from build123d import *

# Parameters (mm, degrees)
SURFACE_EXTRUDE2_1_DEPTH = 115
THICKEN3_T2              = 2
BOSS_EXTRUDE2_REACH      = 890.848
SKETCH11_W               = 70
SKETCH11_H               = 115
BOSS_EXTRUDE7_DEPTH      = 2
SKETCH17_W               = 2.5
SKETCH17_H               = 115
BOSS_EXTRUDE8_DEPTH      = 15
SKETCH22_W               = 1.5
SKETCH22_H               = 105
CUT_EXTRUDE1_DEPTH       = 5
SKETCH23_W               = 64.9
SKETCH23_H               = 2
BOSS_EXTRUDE9_DEPTH      = 15
SKETCH25_W               = 64.9
SKETCH25_H               = 3.5
BOSS_EXTRUDE10_DEPTH     = 15
SKETCH26_W               = 20
SKETCH26_H               = 1.5
CUT_EXTRUDE3_DEPTH       = 15
SKETCH27_W               = 5
SKETCH27_H               = 9
CUT_EXTRUDE4_DEPTH       = 1.1
SKETCH29_W               = 2.5
SKETCH29_H               = 55
CUT_EXTRUDE6_DEPTH       = 1
CUT_EXTRUDE7_REACH       = 905.754
CUT_EXTRUDE7_END_RADIUS  = 63.3
SKETCH30_R               = 2.5
FILLET1_R                = 1
CUT_EXTRUDE8_REACH       = 909.037
SKETCH31_W               = 35
SKETCH31_H               = 3
CUT_EXTRUDE9_REACH       = 905.975
SKETCH32_R               = 1.5
SKETCH33_W               = 1.5
SKETCH33_H               = 5.890969975
BOSS_EXTRUDE11_DEPTH     = 1.5
MIRROR24_COPY_1_REACH    = 905.975
MIRROR24_COPY_1_SKETCH_R = 1.5


with BuildPart() as body_1:
    # Surface-Extrude2: a surface, the sketch's curves swept straight by 115 mm
    with BuildLine(Plane(origin=(0, 0, 0), x_dir=(1, 0, 0), z_dir=(0, 1, 0)), mode=Mode.PRIVATE) as surface_extrude2_1_path:
        ThreePointArc((-880.139667207, 63.554736355), (-845.139667207, 52.580574649), (-810.139667207, 63.554736355))
    surface_extrude2_1 = Shell.extrude(surface_extrude2_1_path.wire(), (0 * SURFACE_EXTRUDE2_1_DEPTH, 1 * SURFACE_EXTRUDE2_1_DEPTH, 0 * SURFACE_EXTRUDE2_1_DEPTH))
    add(Solid.thicken(surface_extrude2_1, -THICKEN3_T2))

    # Sketch11 → Boss-Extrude2 (add, up to next)
    with BuildSketch(Plane(origin=(0, 0, -63.554736355), x_dir=(-1, 0, 0), z_dir=(0, 0, -1)), mode=Mode.PRIVATE) as boss_extrude2_sk1:
        with Locations((845.139667207, 57.5)):
            Rectangle(SKETCH11_W, SKETCH11_H)
    boss_extrude2_tool1 = extrude(boss_extrude2_sk1.sketch, amount=-BOSS_EXTRUDE2_REACH, mode=Mode.PRIVATE) - body_1.part
    add(boss_extrude2_tool1.solids().sort_by_distance((-845.139667, 57.5, -63.554736))[0])

    # Sketch15 → Boss-Extrude7 (add)
    with BuildSketch(Plane(origin=(0, 0, -51.554736355), x_dir=(-1, 0, 0), z_dir=(0, 0, -1))):
        with BuildLine():
            Line((890.139667207, 24.998904399), (845.139667207, 24.998904399))
            Line((845.139667207, 24.998904399), (845.139667207, 15))
            Line((845.139667207, 15), (889.991644173, 15))
            ThreePointArc((889.991644173, 15), (895.139667207, 19.924336912), (890.139667207, 24.998904399))
        make_face()
        with BuildLine():
            Line((891.281592166, 100), (845.139667207, 100))
            Line((845.139667207, 100), (845.139667207, 90.00121851))
            Line((845.139667207, 90.00121851), (891.171212738, 90.00121851))
            ThreePointArc((891.171212738, 90.00121851), (896.281287529, 94.944806923), (891.281592166, 100))
        make_face()
    boss_extrude7 = extrude(amount=BOSS_EXTRUDE7_DEPTH)

    # Mirror20: Boss-Extrude7 across plane
    add(boss_extrude7.mirror(Plane.ZY.offset(845.139667207)))

    # Sketch17 → Boss-Extrude8 (add)
    with BuildSketch(Plane(origin=(0, 0, -63.554736355), x_dir=(-1, 0, 0), z_dir=(0, 0, -1))):
        with Locations((878.889667207, 57.5)):
            Rectangle(SKETCH17_W, SKETCH17_H)
        with Locations((811.489667207, 57.5)):
            Rectangle(SKETCH17_W, SKETCH17_H)
    extrude(amount=BOSS_EXTRUDE8_DEPTH)

    # Sketch22 → Cut-Extrude1 (cut)
    with BuildSketch(Plane(origin=(0, 0, -78.554736355), x_dir=(-1, 0, 0), z_dir=(0, 0, -1))):
        with Locations((811.989667207, 55.5)):
            Rectangle(SKETCH22_W, SKETCH22_H)
    cut_extrude1 = extrude(amount=-CUT_EXTRUDE1_DEPTH, mode=Mode.SUBTRACT)

    # Mirror21: Cut-Extrude1 across plane
    add(cut_extrude1.mirror(Plane.ZY.offset(845.139667207)), mode=Mode.SUBTRACT)

    # Sketch23 → Boss-Extrude9 (add)
    with BuildSketch(Plane(origin=(0, 0, -63.554736355), x_dir=(-1, 0, 0), z_dir=(0, 0, -1))):
        with Locations((845.189667207, 114)):
            Rectangle(SKETCH23_W, SKETCH23_H)
        with Locations((845.189667207, 110)):
            Rectangle(SKETCH23_W, SKETCH23_H)
    extrude(amount=BOSS_EXTRUDE9_DEPTH)

    # Sketch25 → Boss-Extrude10 (add)
    with BuildSketch(Plane(origin=(0, 0, -63.554736355), x_dir=(-1, 0, 0), z_dir=(0, 0, -1))):
        with Locations((845.189667207, 1.75)):
            Rectangle(SKETCH25_W, SKETCH25_H)
    extrude(amount=BOSS_EXTRUDE10_DEPTH)

    # Sketch26 → Cut-Extrude3 (cut)
    with BuildSketch(Plane(origin=(0, 0, -78.554736355), x_dir=(-1, 0, 0), z_dir=(0, 0, -1))):
        with Locations((825.239667207, 1.75)):
            Rectangle(SKETCH26_W, SKETCH26_H)
    extrude(amount=-CUT_EXTRUDE3_DEPTH, mode=Mode.SUBTRACT)

    # Sketch27 → Cut-Extrude4 (cut)
    with BuildSketch(Plane.ZY.offset(880.139667207)):
        with Locations((-75.146974965, 83)):
            Rectangle(SKETCH27_W, SKETCH27_H)
    extrude(amount=-CUT_EXTRUDE4_DEPTH, mode=Mode.SUBTRACT)

    # Sketch29 → Cut-Extrude6 (cut)
    with BuildSketch(Plane(origin=(-810.239667207, 0, 0), x_dir=(0, 0, -1), z_dir=(1, 0, 0))):
        with Locations((77.304736355, 35.5)):
            Rectangle(SKETCH29_W, SKETCH29_H)
    extrude(amount=-CUT_EXTRUDE6_DEPTH, mode=Mode.SUBTRACT)

    # Cut-Extrude7: up to this cylinder (the profile starts inside it)
    cut_extrude7_end = Plane(origin=(-845.139667207, 104, -113.880574649), z_dir=(0, 1, 0)) * Cylinder(CUT_EXTRUDE7_END_RADIUS, 1939.108, mode=Mode.PRIVATE)
    # Sketch30 → Cut-Extrude7 (cut, up to the surface)
    with BuildSketch(Plane(origin=(0, 0, -63.554736355), x_dir=(-1, 0, 0), z_dir=(0, 0, -1)), mode=Mode.PRIVATE) as cut_extrude7_sk1:
        with Locations((822.739667207, 104)):
            Circle(SKETCH30_R)
    cut_extrude7_tool1 = extrude(cut_extrude7_sk1.sketch, amount=-CUT_EXTRUDE7_REACH, mode=Mode.PRIVATE) & cut_extrude7_end
    add(cut_extrude7_tool1.solids().sort_by_distance((-822.739667, 104, -63.554736))[0], mode=Mode.SUBTRACT)

    # Fillet1
    fillet1_edges = [body_1.edges().sort_by_distance(p)[0] for p in [
        (-812.739667207, 3.5, -68.554736355),
        (-812.739667207, 109, -71.054736355),
        (-877.639667207, 109, -71.054736355),
        (-877.639667207, 3.5, -68.554736355),
        (-845.189667207, 3.5, -63.554736355),
        (-812.739667207, 56.25, -63.554736355),
        (-845.189667207, 109, -63.554736355),
        (-877.639667207, 56.25, -63.554736355),
    ]]
    fillet(fillet1_edges, radius=FILLET1_R - 0.0001)  # a hair under: the kernel refuses the full size

    # Sketch31 → Cut-Extrude8 (cut, up to next)
    with BuildSketch(Plane.XZ, mode=Mode.PRIVATE) as cut_extrude8_sk1:
        with Locations((-854.639667207, -77.054736355)):
            Rectangle(SKETCH31_W, SKETCH31_H)
    cut_extrude8_tool1 = extrude(cut_extrude8_sk1.sketch, amount=-CUT_EXTRUDE8_REACH, mode=Mode.PRIVATE) & body_1.part
    add(cut_extrude8_tool1.solids().sort_by_distance((-854.639667, 0, -77.054736))[0], mode=Mode.SUBTRACT)

    # Sketch32 → Cut-Extrude9 (cut, up to next)
    with BuildSketch(Plane(origin=(0, 0, -53.554736355), x_dir=(-1, 0, 0), z_dir=(0, 0, -1)), mode=Mode.PRIVATE) as cut_extrude9_sk1:
        with Locations((889.281592166, 95)):
            Circle(SKETCH32_R)
    cut_extrude9_tool1 = extrude(cut_extrude9_sk1.sketch, amount=-CUT_EXTRUDE9_REACH, mode=Mode.PRIVATE) & body_1.part
    cut_extrude9 = cut_extrude9_tool1.solids().sort_by_distance((-889.281592, 95, -53.554736))[0]
    add(cut_extrude9, mode=Mode.SUBTRACT)

    # Sketch33 → Boss-Extrude11 (add)
    with BuildSketch(Plane.ZY.offset(811.239667207)):
        with Locations((-76.504736355, 105.054515013)):
            Rectangle(SKETCH33_W, SKETCH33_H)
    boss_extrude11 = extrude(amount=BOSS_EXTRUDE11_DEPTH)

    # Mirror22: Boss-Extrude11 across plane
    add(boss_extrude11.mirror(Plane.ZY.offset(845.139667207)))

    # Mirror23: Cut-Extrude9 across plane
    add(cut_extrude9.mirror(Plane.ZY.offset(845.139667207)), mode=Mode.SUBTRACT)

    # Mirror24: Cut-Extrude9 across plane
    add(cut_extrude9.mirror(Plane.ZX.offset(57.5)), mode=Mode.SUBTRACT)

    # Mirror24 copy 1 sketch → Mirror24 copy 1 (cut, up to next)
    with BuildSketch(Plane(origin=(-1690.279334414, 115, -53.554736355), x_dir=(1, 0, 0), z_dir=(0, 0, -1)), mode=Mode.PRIVATE) as mirror24_copy_1_sk1:
        with Locations((889.281592166, 95)):
            Circle(MIRROR24_COPY_1_SKETCH_R)
    mirror24_copy_1_tool1 = extrude(mirror24_copy_1_sk1.sketch, amount=-MIRROR24_COPY_1_REACH, mode=Mode.PRIVATE) & body_1.part
    add(mirror24_copy_1_tool1.solids().sort_by_distance((-800.997742414, 20, -53.554736))[0], mode=Mode.SUBTRACT)


solid = body_1.part
Model file for the job. Use its own axes, mm. A direction names the side the tool comes from. Coordinates: 2 decimals unless noted, no trailing zeros. Order: outer loops, then holes, each group sorted by start corner. A loop starts at its lowest first (then second) coordinate and runs counter-clockwise, first axis right, second up. Notation, with made-up numbers: (12.25, 81) -> (58.25, 81) arc R5 ccw to (58.25, 89) -> close; hole circle Ø5 at (86.25, 77.5). An arc over 180 degrees is marked (long way). Return JSON: item names as keys, results as strings. Group by question number.
Item 1: Pull direction Y, two halves, no side cores. Call faces 4 (the flat face through (-812.74, 56, -68)), 5 (the flat face through (-814, 95, -51.555)), 6 (the flat face through (-879.04, 55, -76)): pulls with the +Y half, pulls with the -Y half, needs draft (parallel to the pull), parting line crosses it, or undercut.
Item 2: Tool access for faces 1 (the flat face through (-872.14, 2, -77)), 2 (the flat face through (-845, 113, -71)), 3 (the cylindrical face through (-887.783, 19.934, -52.569)): list every direction of +Z, -Z, +X, -X, +Y, -Y with a clear straight run to the whole face (end or side of a thin tool).
Item 3: Wall check: line 1 along X through (y, z) = (95, -51.95); line 2 along X through (y, z) = (20, -51.95); line 3 along Y through (x, z) = (-854.5, -70). Give the ranges that are in metal, low to high. Write a range as [from, to].
Item 4: Flat gauge pins, fed straight in: P1, Ø1, axis at y = 86.5, z = -66, coming from the +X side; P2, Ø1.6, axis at x = -868, z = -53, coming from the +Y side; P3, Ø5, axis at y = 19.5, z = -55, coming from the +X side; P4, Ø1.8, axis at x = -889.28, y = 20, coming from the -Z side. Where does each tip first touch, or does it go through?
Item 5: Saw through at C-C on x = -868. Write the cut outline in (y, z), then the cut area to 3 significant figures.
Item 6: Saw through at B-B on z = -66.75. Write the cut outline in (x, y).
Item 7: Saw through at A-A on y = 20. State how many separate pieces and enclosed holes the cut face has, then the cut area to 3 significant figures.
Values found:
{
 "1": {"face 4": "undercut", "face 5": "needs draft", "face 6": "undercut"},
 "2": {"face 1": "-Z, -Y", "face 2": "-Z", "face 3": "+Z, -Z"},
 "3": {"line 1": "x = [-896.28, -890.78], [-887.78, -802.5], [-799.5, -794]", "line 2": "x = [-895.14, -890.78], [-887.78, -802.5], [-799.5, -795.14]", "line 3": "y = [0, 3.5], [109, 111], [113, 115]"},
 "4": {"P1": "stops at x = -810.24", "P2": "stops at y = 100", "P3": "stops at x = -795.14", "P4": "passes through"},
 "5": {"outline": "(0, -75.55) -> (3.5, -75.55) -> (3.5, -64.55) arc R1 cw to (4.5, -63.55) -> (108, -63.55) arc R1 cw to (109, -64.55) -> (109, -78.55) -> (111, -78.55) -> (111, -63.55) -> (113, -63.55) -> (113, -78.55) -> (115, -78.55) -> (115, -54.85) -> (0, -54.85) -> close; (15, -53.55) -> (25, -53.55) -> (25, -51.55) -> (15, -51.55) -> close; (90, -53.55) -> (100, -53.55) -> (100, -51.55) -> (90, -51.55) -> close", "area": "1,140 mm2"},
 "6": {"outline": "(-880.14, 0) -> (-810.24, 0) -> (-810.24, 115) -> (-880.14, 115) -> close; hole (-877.64, 4.5) arc R1 ccw to (-876.64, 3.5) -> (-813.74, 3.5) arc R1 ccw to (-812.74, 4.5) -> (-812.74, 108) arc R1 ccw to (-813.74, 109) -> (-876.64, 109) arc R1 ccw to (-877.64, 108) -> close; hole (-877.64, 111) -> (-812.74, 111) -> (-812.74, 113) -> (-877.64, 113) -> close; hole (-835.24, 1) -> (-815.24, 1) -> (-815.24, 2.5) -> (-835.24, 2.5) -> close"},
 "7": {"separate pieces": "3", "enclosed holes": "0", "area": "858 mm2"}
}
